Model file for the job. Use its own axes, mm. Coordinates: 2 decimals unless noted, no trailing zeros. Order: outer loops, then holes, each group sorted by start corner. A loop starts at its lowest first (then second) coordinate and runs counter-clockwise, first axis right, second up.
from build123d import *

# Parameters (mm, degrees)
F1_DEPTH = 10.37
F5_D     = 12


with BuildPart() as f1:
    # F0 (on Front) → F1 (new body)
    with BuildSketch(Plane.XZ):
        Polygon((9, -5.196152), (9, 5.196152), (0, 10.392305), (-9, 5.196152), (-9, -5.196152), (0, -10.392305), align=None)
    extrude(amount=-F1_DEPTH)

    # F2 (on Right) → F3 (revolve, cut)
    with BuildSketch(Plane.YZ):
        Polygon((0, 14.392305), (0, 9), (3.113249, 14.392305), align=None)
    revolve(axis=Axis((0, 2.79976, 0), (0, 1, 0)), mode=Mode.SUBTRACT)

    # F5 (through all)
    with Locations(Plane.XZ):
        with Locations((0, 0)):
            Hole(F5_D / 2)


solid = f1.part
Q1. Mould opens along Z. For faces 1 (the face through (-0.023, 0.195, 9.338)), 2 (the face through (4.44, 5.11, -7.83)), 3 (the face through (-9, 5, 0)), 4 (the face through (6, 5, 0)) say: pulls with the +Z half, pulls with the -Z half, needs draft (parallel to the pull), parting line crosses it, or undercut.
Established:
face 1: pulls with the +Z half
face 2: pulls with the -Z half
face 3: needs draft
face 4: undercut
Q2. Drop flat-ended pins along their axis: P1, Ø1.5, axis at x = 5.5, y = 2.5, coming from the -Z side; P2, Ø1.5, axis at x = 4, y = 2.5, coming from the -Z side; P3, Ø1.5, axis at x = 6.5, y = 9, coming from the -Z side. Give the stop position or say it passes through.
Established:
P1: stops at z = -7.65
P2: stops at z = -8.52
P3: stops at z = -7.07
Q3. Cut at A-A, the plane y = 4.25. List the corners of the cut face in (x, z).
Established:
outline: (-9, -5.2) - (0, -10.39) - (9, -5.2) - (9, 5.2) - (0, 10.39) - (-9, 5.2) - close; hole circle Ø12 at (0, 0)
Q4. Probe line 1 (Z direction, x = -0.75, y = 10); line 2 (X direction, y = 3.25, z = 1.5); line 3 (Z direction, x = 4.5, y = 5). List the from-to ranges inside material, lowest first.
Established:
line 1: z = -9.96 to -5.95, 5.95 to 9.96
line 2: x = -9 to -5.81, 5.81 to 9
line 3: z = -7.79 to -3.97, 3.97 to 7.79
